Part print with two shaded views. Sizes in mm from the minimum x, y, z corner. Give positions to 0.01 mm unless a question says otherwise; leave off trailing zeros. Order: outer loops, then holes, each group sorted by start corner. A loop starts at its lowest first (then second) coordinate and runs counter-clockwise, first axis right, second up.
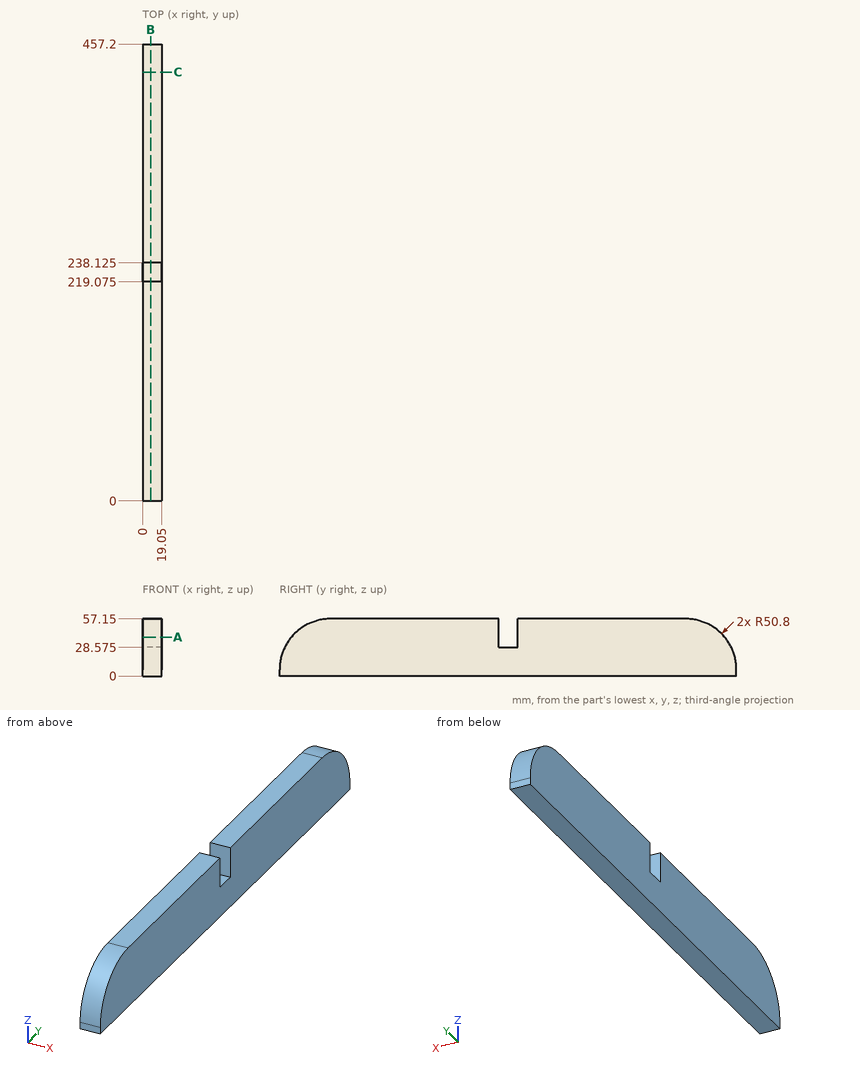
1. Pin check, flat tips, straight feed: P1, Ø5.5, axis at x = 13, z = 49.5, coming from the -Y side; P2, Ø5.5, axis at x = 9.5, z = 37, coming from the +Y side; P3, Ø2, axis at x = 6.5, z = 45, coming from the +Y side. Stop position of each tip, or through.
2. Saw through at A-A on z = 39. Give the cut face in (x, y) (3 decimals).
3. Saw through at C-C on y = 429. Give the cut face in (x, z).
4. Wall check: line 1 (Z direction, x = 7.75, y = 225) (3 decimals); line 2 (Y direction, x = 5.25, z = 9); line 3 (Y direction, x = 12.25, z = 30.5) (3 decimals). Give the ranges that are in metal, low to high.
5. Saw through at B-B on x = 8. Give the cut face in (y, z) (3 decimals), plus the area to 3 significant figures.
Reported:
1. P1: stops at y = 20
1. P2: stops at y = 448.85
1. P3: stops at y = 440.5
2. outline: (0, 11.882) - (19.05, 11.882) - (19.05, 219.075) - (0, 219.075) - close; (0, 238.125) - (19.05, 238.125) - (19.05, 445.318) - (0, 445.318) - close
3. outline: (0, 0) - (19.05, 0) - (19.05, 51.85) - (0, 51.85) - close
4. line 1: z = 0 to 28.575
4. line 2: y = 0.07 to 457.13
4. line 3: y = 6.108 to 219.075, 238.125 to 451.092
5. outline: (0, 0) - (457.2, 0) - (457.2, 6.35) arc R50.8 ccw to (406.4, 57.15) - (238.125, 57.15) - (238.125, 28.575) - (219.075, 28.575) - (219.075, 57.15) - (50.8, 57.15) arc R50.8 ccw to (0, 6.35) - close
5. area: 24,500 mm2
